Answer from the drawing. Dimensions are ordinates in mm from the lowest x, y and z of the part. A direction names the side the tool comes from. Give positions to 0.01 mm unless a question says otherwise; leave off trailing zeros. Order: outer loops, then holes, each group sorted by start corner. A loop starts at its lowest first (then second) coordinate and runs counter-clockwise, first axis right, second up.
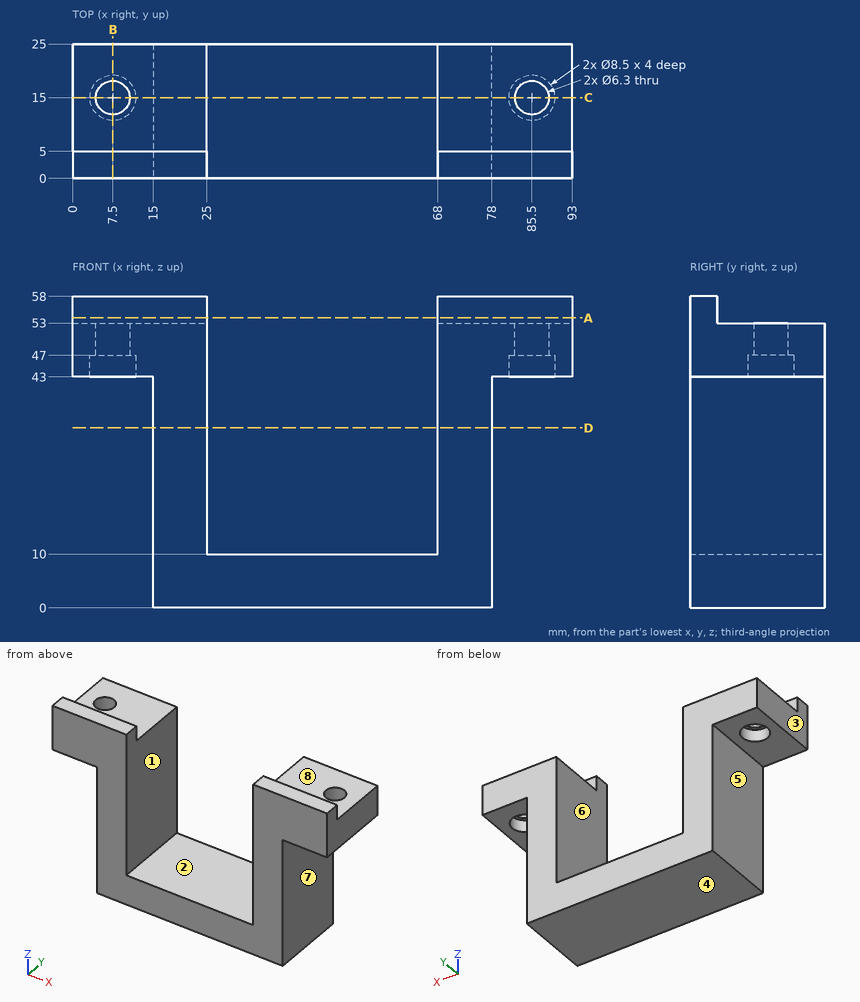
1) The part is cut by section C-C on y = 15. Determine the outline of the cut face in (x, z), and give its area (3 significant figures).
Final values:
outline: (0, 43) - (3.25, 43) - (3.25, 47) - (4.35, 47) - (4.35, 53) - (0, 53) - close; (10.65, 47) - (11.75, 47) - (11.75, 43) - (15, 43) - (15, 0) - (78, 0) - (78, 43) - (81.25, 43) - (81.25, 47) - (82.35, 47) - (82.35, 53) - (68, 53) - (68, 10) - (25, 10) - (25, 53) - (10.65, 53) - close; (88.65, 47) - (89.75, 47) - (89.75, 43) - (93, 43) - (93, 53) - (88.65, 53) - close
area: 1,650 mm2
2) Consider L1, parallel to X at y = 8.75, z = 41.5; L2, parallel to Z at x = 65, y = 23.5; L3, parallel to Y at x = 7.5, z = 44.65. Determine where each line is inside the solid, lowest interval first.
Final values:
L1: x = 15 to 25, 68 to 78
L2: z = 0 to 10
L3: y = 0 to 10.75, 19.25 to 25
3) A tool of negligible diameter and unlimited length cuts with its end or side. For the marked faces 5, 6, 7 and 8, from which of +Z, -Z, +X, -X, +Y, -Y can it reach the whole face along a straight path? Write none if from no direction.
Final values:
face 5: -Z, -X, +Y, -Y
face 6: +Z, +Y, -Y
face 7: -Z, +X, +Y, -Y
face 8: +Z, +X, -X, +Y
4) For a pull along X with two mould halves and no side action, classify the marked faces 1, 2, 3 and 4 as released by +X, released by -X, zero draft, split by the parting line, or undercut.
Final values:
face 1: undercut
face 2: undercut
face 3: released by -X
face 4: zero draft
5) The part is cut by section A-A on z = 54. Determine the outline of the cut face in (x, y).
Final values:
outline: (0, 0) - (25, 0) - (25, 5) - (0, 5) - close; (68, 0) - (93, 0) - (93, 5) - (68, 5) - close
6) Given pin 1 (2 mm diameter, centred on x = 28, y = 10, fed in from +Z); pin 2 (10 mm diameter, centred on x = 7.5, y = 15, fed in from +Z); pin 3 (4.5 mm diameter, centred on x = 83, y = 6.5, fed in from -Z), each flat-ended and moving along its own axis, determine where each tip first touches the part or whether it passes through.
Final values:
pin 1: stops at z = 10
pin 2: stops at z = 53
pin 3: stops at z = 43
7) The part is cut by section D-D on z = 33.5. Determine the outline of the cut face in (x, y).
Final values:
outline: (15, 0) - (25, 0) - (25, 25) - (15, 25) - close; (68, 0) - (78, 0) - (78, 25) - (68, 25) - close
8) The part is cut by section B-B on x = 7.5. Determine the outline of the cut face in (y, z).
Final values:
outline: (0, 43) - (10.75, 43) - (10.75, 47) - (11.85, 47) - (11.85, 53) - (5, 53) - (5, 58) - (0, 58) - close; (18.15, 47) - (19.25, 47) - (19.25, 43) - (25, 43) - (25, 53) - (18.15, 53) - close
